Part model, mm, in its own coordinate system. Give positions to 0.01 mm unless a question says otherwise; leave off trailing zeros.
```python
from build123d import *

# Parameters (mm, degrees)
SKETCH1_W                       = 36.27882
SKETCH1_H                       = 136.0043
EXTRUDE1_DEPTH                  = 6.35
F_3_48_TAPPED_HOLE1_D           = 1.9939
F_3_48_TAPPED_HOLE1_DEPTH       = 9.144
F_3_48_TAPPED_HOLE1_CBORE_D     = 2.5146
F_3_48_TAPPED_HOLE1_CBORE_DEPTH = 7.62
F_3_48_TAPPED_HOLE1_TIP         = 0.599027994


with BuildPart() as part:
    # Sketch1 → Extrude1 (new body)
    with BuildSketch(Plane.XY):
        Rectangle(SKETCH1_W, SKETCH1_H)
    extrude(amount=EXTRUDE1_DEPTH)

    # #3-48 Tapped Hole1
    with Locations(Plane(origin=(-14.071004552, -68.00215, 88.900648793), x_dir=(0, 0, -1), z_dir=(0, -1, 0))):
        with Locations((85.725648793, 25.860414552), (85.725648793, 0.892214552)):
            CounterBoreHole(F_3_48_TAPPED_HOLE1_D / 2, F_3_48_TAPPED_HOLE1_CBORE_D / 2, F_3_48_TAPPED_HOLE1_CBORE_DEPTH, depth=F_3_48_TAPPED_HOLE1_DEPTH)
            with Locations((0, 0, -(F_3_48_TAPPED_HOLE1_DEPTH + F_3_48_TAPPED_HOLE1_TIP / 2))):  # 118° drill point
                Cone(0, F_3_48_TAPPED_HOLE1_D / 2, F_3_48_TAPPED_HOLE1_TIP, mode=Mode.SUBTRACT)


solid = part.part
```
1) Wall check: L1, parallel to X at y = -62, z = 2.25; L2, parallel to Y at x = -13.5, z = 2.5. Give the ranges that are in metal, low to high.
Answers follow:
L1: x = -18.14 to -14.03, -12.33 to 10.94, 12.64 to 18.14
L2: y = -58.71 to 68
2) Two-plate mould, pull along X, no slides. Class faces 1 (the face through (-18.139, -1, 3)), 2 (the face through (12.167, -64.245, 1.976)), 3 (the face through (0, 1, 0)), 4 (the face through (-12.801, -64.245, 1.976)): +X half, -X half, draft (parallel to the pull), parting line (faces both ways), or undercut.
Answers follow:
face 1: -X half
face 2: undercut
face 3: draft
face 4: undercut
3) Pin check, flat tip, straight feed: pin 1 Ø1.6 at (x, z) = (-13.18, 3.17) entering from -Y. Stop position of the tip, or through.
Answers follow:
pin 1: stops at y = -58.74
